Check sheet for the modelled part. Datum: model origin and axes. Units: mm. Round coordinates to 2 decimals unless told otherwise and drop trailing zeros. Write each loop counter-clockwise with the first axis right and the second up, starting at its lowest first coordinate (ties: lowest second). Pieces come first, ordered by that corner, then holes. Notation, with made-up numbers: (43.5, 88.25) -> (60.5, 88.25) arc R35 cw to (60.5, 120.25) -> close; hole circle Ø2 at (-4.75, 3.5). An arc over 180 degrees is marked (long way). One line per item, written item: value. Start each with the question number.
```python
from build123d import *

# Parameters (mm, degrees)
SKETCH1_R           = 3.05
SKETCH1_W           = 89.973098966
SKETCH1_H           = 90.646237781
BOSS_EXTRUDE1_DEPTH = 3.175


with BuildPart() as part:
    # Sketch1 → Boss-Extrude1 (new body)
    with BuildSketch(Plane.XY):
        Polygon((134.366277122, 315.825463089), (134.366277122, 296.898356199), (131.385630367, 296.898356199), (131.385630367, 280.082540759), (135.608213269, 280.082540759), (135.608213269, 277.971249308), (135.608213269, 275.859957857), (131.385630367, 275.859957857), (131.385630367, 259.044142417), (134.366277122, 259.044142417), (134.366277122, 221.189928636), (131.385630367, 221.189928636), (131.385630367, 204.374113196), (135.608213269, 204.374113196), (135.608213269, 202.262821745), (135.608213269, 200.151530294), (131.385630367, 200.151530294), (131.385630367, 183.335714854), (134.366277122, 183.335714854), (134.366277122, 164.408607964), (150.312737258, 164.408607964), (150.312737258, 167.389254718), (167.128552698, 167.389254718), (167.128552698, 173.698290348), (165.63822932, 173.698290348), (165.63822932, 177.126034116), (167.128552698, 177.126034116), (167.128552698, 180.553777884), (171.3511356, 180.553777884), (171.3511356, 177.126034116), (172.841458977, 177.126034116), (172.841458977, 173.698290348), (171.3511356, 173.698290348), (171.3511356, 167.389254718), (188.166951039, 167.389254718), (188.166951039, 164.408607964), (226.021164821, 164.408607964), (226.021164821, 167.389254718), (242.83698026, 167.389254718), (242.83698026, 173.698290348), (241.346656883, 173.698290348), (241.346656883, 177.126034116), (242.83698026, 177.126034116), (242.83698026, 180.553777884), (247.059563162, 180.553777884), (247.059563162, 177.126034116), (248.54988654, 177.126034116), (248.54988654, 173.698290348), (247.059563162, 173.698290348), (247.059563162, 167.389254718), (263.875378602, 167.389254718), (263.875378602, 164.408607964), (279.821838738, 164.408607964), (279.821838738, 183.335714854), (282.802485493, 183.335714854), (282.802485493, 200.151530294), (278.579902591, 200.151530294), (278.579902591, 202.262821745), (278.579902591, 204.374113196), (282.802485493, 204.374113196), (282.802485493, 221.189928636), (279.821838738, 221.189928636), (279.821838738, 259.044142417), (282.802485493, 259.044142417), (282.802485493, 275.859957857), (278.579902591, 275.859957857), (278.579902591, 277.971249308), (278.579902591, 280.082540759), (282.802485493, 280.082540759), (282.802485493, 296.898356199), (279.821838738, 296.898356199), (279.821838738, 315.825463089), (263.875378602, 315.825463089), (263.875378602, 312.844816335), (247.059563162, 312.844816335), (247.059563162, 306.535780705), (248.54988654, 306.535780705), (248.54988654, 303.108036937), (247.059563162, 303.108036937), (247.059563162, 299.680293169), (242.83698026, 299.680293169), (242.83698026, 303.108036937), (241.346656883, 303.108036937), (241.346656883, 306.535780705), (242.83698026, 306.535780705), (242.83698026, 312.844816335), (226.021164821, 312.844816335), (226.021164821, 315.825463089), (188.166951039, 315.825463089), (188.166951039, 312.844816335), (171.3511356, 312.844816335), (171.3511356, 306.535780705), (172.841458977, 306.535780705), (172.841458977, 303.108036937), (171.3511356, 303.108036937), (171.3511356, 299.680293169), (167.128552698, 299.680293169), (167.128552698, 303.108036937), (165.63822932, 303.108036937), (165.63822932, 306.535780705), (167.128552698, 306.535780705), (167.128552698, 312.844816335), (150.312737258, 312.844816335), (150.312737258, 315.825463089), align=None)
        with Locations((157.107508447, 290.442033214)):
            Circle(SKETCH1_R, mode=Mode.SUBTRACT)
        with Locations(Location((256.893063872, 290.685795432, 0), (0, 0, 180))):
            Circle(SKETCH1_R, mode=Mode.SUBTRACT)
        with Locations((257.080607413, 189.795795432)):
            Circle(SKETCH1_R, mode=Mode.SUBTRACT)
        with Locations(Location((157.295282053, 189.548275621, 0), (0, 0, 180))):
            Circle(SKETCH1_R, mode=Mode.SUBTRACT)
        with Locations((207.09405793, 240.117035527)):
            Rectangle(SKETCH1_W, SKETCH1_H, mode=Mode.SUBTRACT)
    extrude(amount=BOSS_EXTRUDE1_DEPTH)


solid = part.part
```
1. Cross-section at C-C (z = 1.05). Give the number of separate pieces and of enclosed holes in the cut face, plus the area to 3 significant figures.
2. Cross-section at B-B (y = 241). Record the cut outline in (x, z) (1 decimal), plus the area to 3 significant figures.
3. Depth check by flat-ended pin: pin 1 Ø1.6 at (y, z) = (310, 2) entering from +X; pin 2 Ø1 at (x, z) = (159.5, 2) entering from -Y; pin 3 Ø1 at (y, z) = (304.5, 1.5) entering from -X; pin 4 Ø8 at (x, y) = (168.5, 249) entering from +Z. Enter the tip coordinate at first touch or a pass-through.
4. Cross-section at A-A (x = 229.5). Record the cut outline in (y, z) (3 decimals), plus the area to 3 significant figures.
5. Material ranges on probe 1 along X at (y, z) = (303, 1); probe 2 along X at (y, z) = (203, 1.9); probe 3 along X at (y, z) = (262, 2.9), recorded low to high.
6. Release check for a two-part mould opening along Y. For faces 1 (the face through (206, 292, 3.175)), 2 (the face through (254.833, 191.857, 1.565)) record: +Y half, -Y half, draft (parallel to the pull), parting line (faces both ways), or undercut.
Working result:
1. separate pieces: 1
1. enclosed holes: 5
1. area: 13,400 mm^2
2. outline: (134.4, 0) -> (162.1, 0) -> (162.1, 3.2) -> (134.4, 3.2) -> close; (252.1, 0) -> (279.8, 0) -> (279.8, 3.2) -> (252.1, 3.2) -> close
2. area: 176 mm^2
3. pin 1: stops at x = 279.82
3. pin 2: stops at y = 167.39
3. pin 3: stops at x = 134.37
3. pin 4: passes through
4. outline: (167.389, 0) -> (194.794, 0) -> (194.794, 3.175) -> (167.389, 3.175) -> close; (285.44, 0) -> (312.845, 0) -> (312.845, 3.175) -> (285.44, 3.175) -> close
4. area: 174 mm^2
5. probe 1: x = 134.37 to 167.13, 171.35 to 242.84, 247.06 to 279.82
5. probe 2: x = 135.61 to 162.11, 252.08 to 278.58
5. probe 3: x = 131.39 to 162.11, 252.08 to 282.8
6. face 1: draft
6. face 2: undercut
